Autodesk Inventor part; units mm, degrees
ref_plane "YZ Plane" through (0, 0, 0) normal (1, 0, 0) x (0, 1, 0)
ref_plane "XZ Plane" through (0, 0, 0) normal (0, 1, 0) x (-1, 0, 0)
ref_plane "XY Plane" through (0, 0, 0) normal (0, 0, 1) x (1, 0, 0)
sketch "Sketch1" plane through (0, 0, 0) normal (0, 1, 0) x (-1, 0, 0)
  circle A0 centre (0, 0) radius 25
  dimension "d0" = 50
extrude "Extrusion1" add sketch "Sketch1" along normal blind 80
sketch "Sketch2" plane through (0, 80, 0) normal (0, 1, 0) x (1, 0, 0)
  circle A0 centre (0, 0) radius 10
  circle A1 centre (0, 0) radius 2.5
  dimension "d3" = 20
  dimension "d4" = 5
extrude "Extrusion2" add sketch "Sketch2" along normal blind 2 contours A0 | A1
extrude "Extrusion3" add sketch "Sketch2" along normal blind 30 contours A1
fillet "Fillet1" radius 2 3 edges at (25, 0, 0) (25, 80, 0) (-10, 82, 0)
fillet "Fillet2" radius 1 1 edges at (-2.5, 110, 0)
properties part number "Motor DC" material "Stainless Steel, Brushed"
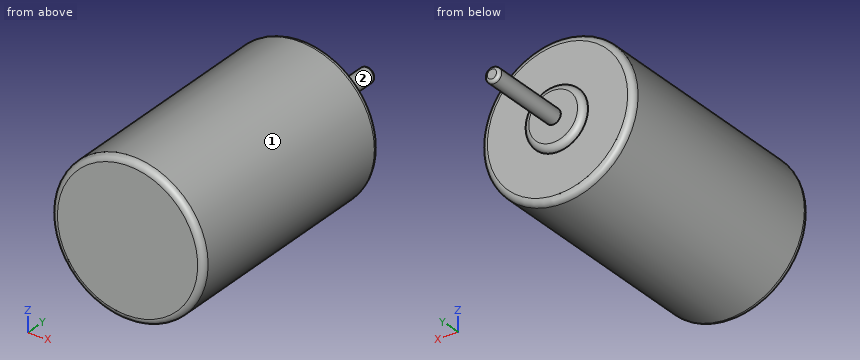
CAD build for the part. Positions are in the model's coordinates, mm. Face numbers are marked on the shaded views. A direction names the side the tool comes from. Give positions to 0.01 mm unless a question says otherwise; leave off trailing zeros. Write each loop counter-clockwise with the first axis right and the second up, starting at its lowest first coordinate (ties: lowest second). Pieces come first, ordered by that corner, then holes. Notation, with made-up numbers: M -23.5,-38.75 L 15.5,-38.75 A19 ccw 15.5,-3.75 Z; hole C 1,35 d1. An arc over 180 degrees is marked long. Put each result on its own line as item: value. Start each with the question number.
(1) Flat gauge pins, fed straight in: pin 1 Ø6 at (x, y) = (8, 17.5) entering from -Z; pin 2 Ø3 at (y, z) = (62.5, 17.5) entering from -X; pin 3 Ø1.5 at (x, y) = (2, 28) entering from -Z. Where does each tip first touch, or does it go through?
(2) Which spindle directions (+Z, -Z, +X, -X, +Y, -Y) get a long thin tool onto all of the face, cutting with end or side? Do the marked faces 1 and 2. Say none if no direction does.
(3) Band-saw the part on C-C, the plane y = 18. Write the cut outline in (x, z).
(4) Probe L1, parallel to Y at x = 17.5, z = -10; L2, parallel to X at y = 36.5, z = 0.5 (3 decimals); L3, parallel to Y at x = 7, z = -2. List the from-to ranges inside material, lowest first.
Response values:
1. pin 1: stops at z = -24.49
1. pin 2: stops at x = -19.21
1. pin 3: stops at z = -24.97
2. face 1: +Y, -Y
2. face 2: +Y
3. outline: C 0,0 d50
4. L1: y = 0 to 80
4. L2: x = -24.995 to 24.995
4. L3: y = 0 to 82
